from build123d import *

# Parameters (mm, degrees)
SKETCH1_W                                 = 75
SKETCH1_H                                 = 55
BOSS_EXTRUDE1_DEPTH                       = 10
M2_5X0_45_TAPPED_HOLE1_OUTLINE_R          = 1.025
M2_5X0_45_TAPPED_HOLE1_DEPTH              = 10
CSK_FOR_8_FLAT_HEAD_MACHINE_SCREW_2_COUNT = 2
CSK_FOR_8_FLAT_HEAD_MACHINE_SCREW_2_PITCH = 30
FILLET1_R                                 = 3
CHAMFER1_SIZE                             = 1


# Read off the part's stored shape, not the designer's step: M2.5x0.45 Tapped Hole1
with BuildPart() as part:
    # Sketch1 → Boss-Extrude1 (new body)
    with BuildSketch(Plane(origin=(0, 0, 0), x_dir=(1, 0, 0), z_dir=(0, 1, 0))):
        Rectangle(SKETCH1_W, SKETCH1_H)
    extrude(amount=BOSS_EXTRUDE1_DEPTH)

    # M2.5x0.45 Tapped Hole1 outline → M2.5x0.45 Tapped Hole1 (cut)
    with BuildSketch(Plane(origin=(0, 0, 0), x_dir=(1, 0, 0), z_dir=(0, 1, 0))):
        with Locations((33, -23)):
            Circle(M2_5X0_45_TAPPED_HOLE1_OUTLINE_R)
        with Locations((-33, 23)):
            Circle(M2_5X0_45_TAPPED_HOLE1_OUTLINE_R)
        with Locations((-33, -23)):
            Circle(M2_5X0_45_TAPPED_HOLE1_OUTLINE_R)
        with Locations((33, 23)):
            Circle(M2_5X0_45_TAPPED_HOLE1_OUTLINE_R)
    extrude(amount=M2_5X0_45_TAPPED_HOLE1_DEPTH, mode=Mode.SUBTRACT)

    # Sketch6 → CSK for #8 Flat Head Machine Screw (100)1 (revolve, cut)
    with BuildSketch(Plane(origin=(15, 10, 0), x_dir=(0, 0, 1), z_dir=(1, 0, 0))):
        Polygon((0, 0), (0, 10), (2.2479, 10), (2.2479, 7.651759845), (4.216390729, 6), (4.216390729, 0), align=None)
    csk_for_8_flat_head_machine_screw_100 = revolve(axis=Axis((15, 16.35, 0), (0, -1, 0)), mode=Mode.SUBTRACT)

    # CSK for _8 Flat Head Machine Screw _ 2: CSK for #8 Flat Head Machine Screw (100)1 ×2
    with Locations(*[(-i * CSK_FOR_8_FLAT_HEAD_MACHINE_SCREW_2_PITCH, 0, 0) for i in range(1, CSK_FOR_8_FLAT_HEAD_MACHINE_SCREW_2_COUNT)]):
        add(csk_for_8_flat_head_machine_screw_100, mode=Mode.SUBTRACT)

    # Fillet1
    fillet1_edges = [part.edges().sort_by_distance(p)[0] for p in [
        (37.5, 5, 27.5),
        (-37.5, 5, 27.5),
        (-37.5, 5, -27.5),
        (37.5, 5, -27.5),
    ]]
    fillet(fillet1_edges, radius=FILLET1_R)

    # Chamfer1
    chamfer1_edges = [part.edges().sort_by_distance(p)[0] for p in [
        (37.5, 0, 0),
        (37.5, 10, 0),
        (0, 0, 27.5),
        (-37.5, 0, 0),
        (0, 0, -27.5),
        (-36.621320344, 0, 26.621320344),
        (36.621320344, 0, -26.621320344),
        (-36.621320344, 0, -26.621320344),
        (36.621320344, 0, 26.621320344),
        (0, 10, 27.5),
        (0, 10, -27.5),
        (-37.5, 10, 0),
        (-36.621320344, 10, 26.621320344),
        (36.621320344, 10, -26.621320344),
        (-36.621320344, 10, -26.621320344),
        (36.621320344, 10, 26.621320344),
    ]]
    chamfer(chamfer1_edges, length=CHAMFER1_SIZE)


solid = part.part
Source: CAD feature listing. Evaluate the final solid. Frame: model axes, mm. Round coordinates to 2 decimals unless told otherwise and drop trailing zeros. Loops run counter-clockwise (first coordinate to the right, second up) from the corner with the lowest first, then second, coordinate; pieces in that order, holes last. Notation, with made-up numbers: (66.5, 40) - (118.5, 40) arc R17 ccw to (118.5, 70) - close; hole circle Ø8 at (62, -27). An arc over 180 degrees is marked (long way). Write item = value, one per line. Start each with the question number.
(1) Ray query, line 1 along Z through (x, y) = (-33, 3) (3 decimals); line 2 along X through (y, z) = (6, 23) (3 decimals); line 3 along X through (y, z) = (5.5, 0). Return the intervals inside material, ascending. Write a range as from..to.
(2) Pin query (flat end, axial travel): pin 1 (9.5 mm diameter, centred on x = 15, z = 0, fed in from -Y); pin 2 (6.5 mm diameter, centred on x = -15, z = 0, fed in from +Y). Return the tip coordinate at first contact, or that it passes through.
(3) Section query A-A, the plane x = -33. Output: boundary loops of the cut face in (y, z) (3 decimals), plus the area to 3 significant figures.
(4) Pull-direction query (X, two-part tool) for faces 1 (the face through (36.21, 9.6, -26.18)), 2 (the face through (-36.18, 0.4, -26.21)), 3 (the face through (10.82, 7.04, -0.55)); classes: +X half, -X half, draft (parallel to the pull), parting line (faces both ways), or undercut.
(5) Section query C-C, the plane y = 7.5. Output: boundary loops of the cut face in (x, z) (3 decimals).
(6) Section query D-D, the plane x = 15. Output: boundary loops of the cut face in (y, z), plus the area to 3 significant figures.
(7) Section query B-B, the plane z = 0. Output: boundary loops of the cut face in (x, y).
Conclusion:
q1.line_1 = -27.5..-24.025, -21.975..21.975, 24.025..27.5
q1.line_2 = -37.5..-34.025, -31.975..31.975, 34.025..37.5
q1.line_3 = -37.5..-19.22, -10.78..10.78, 19.22..37.5
q2.pin_1 = 0
q2.pin_2 = 3.19
q3.outline = (0, -26.5) - (1, -27.5) - (9, -27.5) - (10, -26.5) - (10, -24.025) - (0, -24.025) - close; (0, -21.975) - (10, -21.975) - (10, 21.975) - (0, 21.975) - close; (0, 24.025) - (10, 24.025) - (10, 26.5) - (9, 27.5) - (1, 27.5) - (0, 26.5) - close
q3.area = 507 mm2
q4.face_1 = +X half
q4.face_2 = -X half
q4.face_3 = undercut
q5.outline = (-37.5, -24.5) arc R3 ccw to (-34.5, -27.5) - (34.5, -27.5) arc R3 ccw to (37.5, -24.5) - (37.5, 24.5) arc R3 ccw to (34.5, 27.5) - (-34.5, 27.5) arc R3 ccw to (-37.5, 24.5) - close; hole circle Ø2.05 at (-33, -23); hole circle Ø2.05 at (-33, 23); hole circle Ø8.433 at (-15, 0); hole circle Ø8.433 at (15, 0); hole circle Ø2.05 at (33, -23); hole circle Ø2.05 at (33, 23)
q6.outline = (0, -26.5) - (1, -27.5) - (9, -27.5) - (10, -26.5) - (10, -4.22) - (4, -4.22) - (2.35, -2.25) - (0, -2.25) - close; (0, 2.25) - (2.35, 2.25) - (4, 4.22) - (10, 4.22) - (10, 26.5) - (9, 27.5) - (1, 27.5) - (0, 26.5) - close
q6.area = 476 mm2
q7.outline = (-37.5, 1) - (-36.5, 0) - (-17.25, 0) - (-17.25, 2.35) - (-19.22, 4) - (-19.22, 10) - (-36.5, 10) - (-37.5, 9) - close; (-12.75, 0) - (12.75, 0) - (12.75, 2.35) - (10.78, 4) - (10.78, 10) - (-10.78, 10) - (-10.78, 4) - (-12.75, 2.35) - close; (17.25, 0) - (36.5, 0) - (37.5, 1) - (37.5, 9) - (36.5, 10) - (19.22, 10) - (19.22, 4) - (17.25, 2.35) - close
